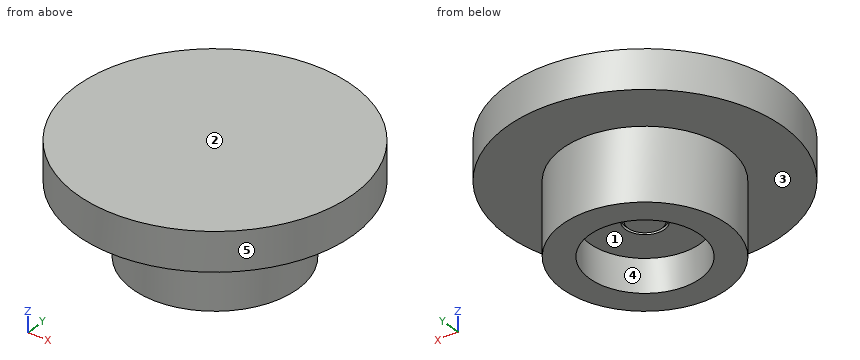
Autodesk Fusion 360 part; units mm, degrees
sketch "Sketch1" plane through (0, 0, 0) normal (0, 0, 1) x (1, 0, 0)
  circle A0 centre (0, 0) radius 14.95
  circle A1 centre (0, 0) radius 10.05
  circle A2 centre (0, 0) radius 3.05
  circle A3 centre (0, 0) radius 3.55
  circle A4 centre (0, 0) radius 25
  dimension "d1" = 29.9
  dimension "d2" = 20.1
  dimension "d7" = 6.1
  dimension "d8" = 7.1
  dimension "d9" = 50
extrude "Extrude1" add sketch "Sketch1" against normal blind 13 contours A0
extrude "Extrude2" add sketch "Sketch1" against normal blind 7 contours A1 | A2 | A3
extrude "Extrude3" add sketch "Sketch1" against normal blind 8 contours A3
extrude "Extrude4" cut 1 faces at (3.3701, -0.1764, -8) along direction (0, 0, 1) blind 1.5
extrude "Extrude5" add sketch "Sketch1" along normal blind 7 contours A0 | A1 | A2 | A3 | A4
Work out the finished part from the listing and answer in its coordinate system (mm). Face numbers are marked on the shaded views. A direction names the side the tool comes from. Round coordinates to 2 decimals unless told otherwise and drop trailing zeros. Write each loop counter-clockwise with the first axis right and the second up, starting at its lowest first coordinate (ties: lowest second). Pieces come first, ordered by that corner, then holes. Notation, with made-up numbers: (50.25, 7.25) - (98.25, 7.25) arc R12 ccw to (98.25, 24.25) - close; hole circle Ø7 at (46, 12.25). An arc over 180 degrees is marked (long way). Return JSON: item names as keys, results as strings. Group by question number.
Q1. For the marked faces 1 and 2, determine the directions among +Z, -Z, +X, -X, +Y, -Y from which every point of the face is accessible in a straight line to the end or side of a thin tool.
Q2. The mould has two halves that part along Y. Classify the marked faces 3, 4 and 5: released by +Y, released by -Y, zero draft, split by the parting line, or undercut.
Q3. Find the intervals of material crossed by L1, parallel to Y at x = 0, z = -6.85; L2, parallel to Z at x = 15, y = 4; L3, parallel to Y at x = 0, z = -8.7, in increasing order.
Q4. The part is cut by section A-A on x = -6. Write down the section's boundary in (y, z).
Q5. The part is cut by section D-D on z = 1.25. Write down the section's boundary in (x, y), then the cut area to 3 significant figures.
Q6. Each of these flat-tipped pins is pushed along its axis until it touches: pin 1 Ø1.5 at (x, z) = (13.5, -8) entering from +Y; pin 2 Ø10 at (x, z) = (-0.5, -4) entering from +Y; pin 3 Ø4 at (x, z) = (5.5, -11) entering from +Y. Where does it stop, or does it pass through?
Q7. The part is cut by section B-B on y = 9. Write down the section's boundary in (x, z).
Q8. The part is cut by section C-C on z = -10. Write down the section's boundary in (x, y).
Solved:
{
 "1": {"face 1": "-Z", "face 2": "+Z, +X, -X, +Y, -Y"},
 "2": {"face 3": "zero draft", "face 4": "undercut", "face 5": "split by the parting line"},
 "3": {"L1": "-14.95 to -3.55, -3.05 to 3.05, 3.55 to 14.95", "L2": "0 to 7", "L3": "-14.95 to -10.05, 10.05 to 14.95"},
 "4": {"outline": "(-24.27, 0) - (-13.69, 0) - (-13.69, -13) - (-8.06, -13) - (-8.06, -7) - (8.06, -7) - (8.06, -13) - (13.69, -13) - (13.69, 0) - (24.27, 0) - (24.27, 7) - (-24.27, 7) - close"},
 "5": {"outline": "circle Ø50 at (0, 0)", "area": "1,960 mm²"},
 "6": {"pin 1": "y = 7.81", "pin 2": "y = 25", "pin 3": "y = 14.53"},
 "7": {"outline": "(-23.32, 0) - (-11.94, 0) - (-11.94, -13) - (-4.47, -13) - (-4.47, -7) - (4.47, -7) - (4.47, -13) - (11.94, -13) - (11.94, 0) - (23.32, 0) - (23.32, 7) - (-23.32, 7) - close"},
 "8": {"outline": "circle Ø29.9 at (0, 0); hole circle Ø20.1 at (0, 0)"}
}
